Autodesk Inventor part; units mm, degrees
ref_plane "YZ Plane" through (0, 0, 0) normal (1, 0, 0) x (0, 1, 0)
ref_plane "XZ Plane" through (0, 0, 0) normal (0, 1, 0) x (-1, 0, 0)
ref_plane "XY Plane" through (0, 0, 0) normal (0, 0, 1) x (1, 0, 0)
sketch "草图1" plane through (0, 0, 0) normal (0, 0, 1) x (1, 0, 0)
  circle A0 centre (0, 0) radius 4
  dimension "d0" = 8
extrude "拉伸1" add sketch "草图1" along normal blind 1
sketch "草图2" plane through (0, 0, 1) normal (0, 0, 1) x (1, 0, 0)
  line L0 (1.4434, -2.5) -> (-1.4434, -2.5)
  line L1 (-1.4434, -2.5) -> (-2.8868, 0)
  line L2 (-2.8868, 0) -> (-1.4434, 2.5)
  line L3 (-1.4434, 2.5) -> (1.4434, 2.5)
  line L4 (1.4434, 2.5) -> (2.8868, 0)
  line L5 (2.8868, 0) -> (1.4434, -2.5)
  line L6 (0, 0) -> (0, 2.5)
  dimension "d3" = 5
extrude "拉伸2" add sketch "草图2" along normal blind 4
sketch "草图3" plane through (0, 0, 0) normal (0, 0, -1) x (-1, 0, 0)
  circle A0 centre (0, 0) radius 2.5
  dimension "d6" = 5
extrude "拉伸3" add sketch "草图3" along normal blind 19
thread "螺纹1"
chamfer "倒角1" distance 0.25 angle 45 1 edges at (2.5, 0, -19)
properties part number "电机座上轴盖固定螺丝"
Could you check a few things on this model? Use its own coordinates, in mm. A direction names the side the tool comes from. Coordinates: 2 decimals unless noted, no trailing zeros. Loops run counter-clockwise (first coordinate to the right, second up) from the corner with the lowest first, then second, coordinate; pieces in that order, holes last.
1. For P1, Ø1.4, axis at x = 0.5, z = 3.5, coming from the +Y side; P2, Ø4, axis at x = -2, z = -11.5, coming from the -Y side; P3, Ø1, axis at y = 1.5, z = -6, coming from the +X side, each with a flat end and sliding along its axis, tell me the tip position at first contact or that it passes through.
2. I need wall thicknesses on L1, parallel to Z at x = 2.25, y = 3; L2, parallel to Y at x = 0.5, z = -1.75; L3, parallel to Y at x = 2.25, z = -9.25. Which ranges of each line are inside material? Lowest first, please.
3. Imagine slicing it at A-A (x = 0). Please give me the cut outline in (y, z), and give its area (3 significant figures).
4. Imagine slicing it at C-C (x = -3.5). Please give me the cut outline in (y, z), and give its area (3 significant figures).
5. Imagine slicing it at B-B (z = -17.5). Please give me the cut outline in (x, y), and give its area (3 significant figures).
6. For faces 1 (the face through (0, 2.5, 3)), 2 (the face through (-2.175, 1.233, 2.972)), 3 (the face through (2.155, 1.267, 2.972)), 4 (the face through (2.175, -1.233, 2.972)), 5 (the face through (0.54, 2.44, -9.24)), which set-ups out of +Z, -Z, +X, -X, +Y, -Y let a thin tool reach every point of the face, with its end or its side?
Computed values:
1. P1: stops at y = 2.5
1. P2: stops at y = -2.5
1. P3: stops at x = 2.29
2. L1: z = 0 to 1
2. L2: y = -2.45 to 2.45
2. L3: y = -1.09 to 1.09
3. outline: (-4, 0) - (-2.5, 0) - (-2.5, -18.75) - (-2.25, -19) - (2.25, -19) - (2.5, -18.75) - (2.5, 0) - (4, 0) - (4, 1) - (2.5, 1) - (2.5, 5) - (-2.5, 5) - (-2.5, 1) - (-4, 1) - close
3. area: 123 mm2
4. outline: (-1.94, 0) - (1.94, 0) - (1.94, 1) - (-1.94, 1) - close
4. area: 3.87 mm2
5. outline: circle Ø5 at (0, 0)
5. area: 19.6 mm2
6. face 1: +Z, +X, -X, +Y
6. face 2: +Z, -X, +Y
6. face 3: +Z, +X, +Y
6. face 4: +Z, +X, -Y
6. face 5: -Z
